Work out the finished part from the listing and answer in its coordinate system (mm). A direction names the side the tool comes from. Give positions to 0.01 mm unless a question says otherwise; leave off trailing zeros. Write each loop counter-clockwise with the first axis right and the second up, starting at its lowest first coordinate (ties: lowest second). Pieces come first, ordered by that corner, then holes.
1) Straight lines are drawn through the part: probe 1 along X at (y, z) = (9.5, 5.2); probe 2 along Y at (x, z) = (11.5, 0.45). For each, find the intervals that lie inside material, in ascending order.
2) Find section A-A (y = -9.5). Determine the outline of the cut face in (x, z).
3) Find section B-B (z = 2.35). Determine the outline of the cut face in (x, y), plus the area to 3 significant figures.
4) A tool of negligible diameter and unlimited length cuts with its end or side. For faces 1 (the face through (5, -21, 3)), 2 (the face through (11.7, -4, 3)), from which of +Z, -Z, +X, -X, +Y, -Y can it reach the whole face along a straight path? Write none if from no direction.
5) Determine the mould class of faces 3 (the face through (10, 14, 3)), 4 (the face through (0, 21, 3)), 5 (the face through (17.5, 0, 3)) for opening direction X: pulls with the +X half, pulls with the -X half, needs draft (parallel to the pull), parting line crosses it, or undercut.
6) Given pin 1 Ø12 at (x, y) = (-3.5, -15.5) entering from -Z; pin 2 Ø2 at (x, z) = (9, 4) entering from -Y, each flat-ended and moving along its own axis, determine where each tip first touches the part or whether it passes through.
```python
from build123d import *

# Parameters (mm, degrees)
ESQUISSE1_W             = 35
ESQUISSE1_H             = 42
BOSS_EXTRU_1_DEPTH      = 6
ESQUISSE2_W             = 4
ESQUISSE2_H             = 35
ESQUISSE2_W_2           = 3.5
ENL_V_MAT_EXTRU_1_DEPTH = 6


with BuildPart() as part:
    # Esquisse1 → Boss.-Extru.1 (new body)
    with BuildSketch(Plane.XY):
        Rectangle(ESQUISSE1_W, ESQUISSE1_H)
    extrude(amount=BOSS_EXTRU_1_DEPTH)

    # Esquisse2 → Enlèv. mat.-Extru.1 (cut)
    with BuildSketch(Plane(origin=(0, 0, 0), x_dir=(-1, 0, 0), z_dir=(0, 0, -1))):
        with Locations((-9.7, -3.5)):
            Rectangle(ESQUISSE2_W, ESQUISSE2_H)
        with Locations((9.7, -3.5)):
            Rectangle(ESQUISSE2_W, ESQUISSE2_H)
        with Locations((0, -3.5)):
            Rectangle(ESQUISSE2_W_2, ESQUISSE2_H)
    extrude(amount=-ENL_V_MAT_EXTRU_1_DEPTH, mode=Mode.SUBTRACT)


solid = part.part
```
Results:
1. probe 1: x = -17.5 to -11.7, -7.7 to -1.75, 1.75 to 7.7, 11.7 to 17.5
1. probe 2: y = 14 to 21
2. outline: (-17.5, 0) - (-11.7, 0) - (-11.7, 6) - (-17.5, 6) - close; (-7.7, 0) - (-1.75, 0) - (-1.75, 6) - (-7.7, 6) - close; (1.75, 0) - (7.7, 0) - (7.7, 6) - (1.75, 6) - close; (11.7, 0) - (17.5, 0) - (17.5, 6) - (11.7, 6) - close
3. outline: (-17.5, -21) - (-11.7, -21) - (-11.7, 14) - (-7.7, 14) - (-7.7, -21) - (-1.75, -21) - (-1.75, 14) - (1.75, 14) - (1.75, -21) - (7.7, -21) - (7.7, 14) - (11.7, 14) - (11.7, -21) - (17.5, -21) - (17.5, 21) - (-17.5, 21) - close
3. area: 1,070 mm2
4. face 1: +Z, -Z, +X, -X, -Y
4. face 2: +Z, -Z, -Y
5. face 3: undercut
5. face 4: needs draft
5. face 5: pulls with the +X half
6. pin 1: stops at z = 0
6. pin 2: stops at y = 14
